Autodesk Inventor part; units mm, degrees
ref_plane "YZ Plane" through (0, 0, 0) normal (1, 0, 0) x (0, 1, 0)
ref_plane "XZ Plane" through (0, 0, 0) normal (0, 1, 0) x (-1, 0, 0)
ref_plane "XY Plane" through (0, 0, 0) normal (0, 0, 1) x (1, 0, 0)
sketch "Sketch1" plane through (0, 0, 0) normal (0, 0, 1) x (1, 0, 0)
  circle A0 centre (0, 0) radius 20
  circle A1 centre (0, 0) radius 23
  dimension "d0" = 40
  dimension "d1" = 46
extrude "Extrusion1" add sketch "Sketch1" along normal mid plane 520
sketch "Sketch2" plane through (0, 0, 0) normal (1, 0, 0) x (0, 1, 0)
  line L0 (0, 280) -> (0, -280)
  line L1 (-280, 0) -> (280, 0)
  point P0 (0, 0)
  point P1 (0, 200)
  point P2 (0, 0)
  point P3 (0, -200)
  dimension "d4" = 200
  dimension "d5" = 200
hole "Hole1" at (0, 0, 200) at (0, 0, 0) at (0, 0, -200) direction (-1, 0, 0) diameter 4.5 end through all
sketch "Sketch3" plane through (0, 0, 0) normal (1, 0, 0) x (0, 1, 0)
  line L0 (23, -240) -> (7, -240)
  line L1 (7, -240) -> (7, 240)
  line L2 (7, 240) -> (23, 240)
  line L3 (23, 240) -> (23, -240)
  line L4 (23, 260) -> (-23, 260)
  line L5 (-23, -260) -> (23, -260)
  line L6 (0, 350) -> (0, -350)
  point P0 (0, 0)
  dimension "d13" = 20
  dimension "d14" = 20
  dimension "d15" = 7
extrude "Extrusion2" cut sketch "Sketch3" along normal through all both and the other way through all
fillet "Fillet1" radius 2 4 edges at (20.3219, 7, -240) (-20.3219, 7, -240) (20.3219, 7, 240) (-20.3219, 7, 240)
properties part number "Pancake_Tilt Pipe" material "PVC-Piping"
For this review, take the finished solid that the model builds, in its own axes (mm). A direction names the side the tool comes from. Give positions to 0.01 mm unless a question says otherwise; leave off trailing zeros. Loops run counter-clockwise (first coordinate to the right, second up) from the corner with the lowest first, then second, coordinate; pieces in that order, holes last. Notation, with made-up numbers: (10.25, -30.5) - (43.25, -30.5) arc R19 cw to (43.25, 4.5) - close; hole circle Ø10 at (65.25, 58). An arc over 180 degrees is marked (long way). Write each question's results on one line, items separated by ' | '.
(1) Take a section at D-D (z = 215.5). Give the boundary of the cut face in (x, y) (3 decimals), then the cut area to 3 significant figures.
Conclusion:
outline: (-21.909, 7) arc R23 ccw (long way) to (21.909, 7) - (18.735, 7) arc R20 cw (long way) to (-18.735, 7) - close | area: 245 mm^2
(2) Draft analysis for pull direction X (two halves, no side actions). For faces 1 (the cylindrical face through (-4.336, -19.524, 3.64)), 2 (the flat face through (-7, 19, -260)), 3 (the cylindrical face through (-2.994, -22.804, -3.64)), state which applies: +X half, -X half, draft (parallel to the pull), parting line (faces both ways), or undercut.
Conclusion:
face 1: undercut | face 2: draft | face 3: parting line
(3) Take a section at C-C (y = -10). Give the boundary of the cut face in (x, z), then the cut area to 3 significant figures.
Conclusion:
outline: (-20.71, -260) - (-17.32, -260) - (-17.32, 260) - (-20.71, 260) - close; (17.32, -260) - (20.71, -260) - (20.71, 260) - (17.32, 260) - close | area: 3,530 mm^2
(4) For pin 1 Ø1 at (x, z) = (-21, 16) entering from +Y; pin 2 Ø7 at (x, y) = (-9.5, 12.5) entering from -Z; pin 3 Ø12 at (x, z) = (2.5, -156.5) entering from +Y; pin 4 Ø3 at (x, z) = (-17, 75.5) entering from +Y, all flat-tipped, find the tip position at first contact; note any pin that passes through.
Conclusion:
pin 1: y = 7 | pin 2: through | pin 3: y = -18.1 | pin 4: y = -7.6
(5) Take a section at B-B (y = 14.5). Give the boundary of the cut face in (x, z), then the cut area to 3 significant figures.
Conclusion:
outline: (-17.85, -260) - (-13.77, -260) - (-13.77, -240) - (-17.85, -240) - close; (-17.85, 240) - (-13.77, 240) - (-13.77, 260) - (-17.85, 260) - close; (13.77, -260) - (17.85, -260) - (17.85, -240) - (13.77, -240) - close; (13.77, 240) - (17.85, 240) - (17.85, 260) - (13.77, 260) - close | area: 326 mm^2
(6) Take a section at A-A (x = 0). Give the boundary of the cut face in (y, z), then the cut area to 3 significant figures.
Conclusion:
outline: (-23, -260) - (-20, -260) - (-20, 260) - (-23, 260) - close; (20, -260) - (23, -260) - (23, -240) - (20, -240) - close; (20, 240) - (23, 240) - (23, 260) - (20, 260) - close | area: 1,680 mm^2
(7) For line 1 along X through (y, z) = (-0.5, 62); line 2 along Z through (x, y) = (6.5, 19); line 3 along X through (y, z) = (-9, -42), list the stretches that pass through material, from the lowest coordinate up.
Conclusion:
line 1: -22.99 to -19.99, 19.99 to 22.99 | line 2: -260 to -240, 240 to 260 | line 3: -21.17 to -17.86, 17.86 to 21.17
(8) For faces 4 (the flat face through (-1.7, 20.1, 240)), 5 (the flat face through (-7, 19, 260)), list the 3-axis set-ups (+Z, -Z, +X, -X, +Y, -Y) from which the entire face can be reached by the end or side of a thin tool; tool diameter is ignored.
Conclusion:
face 4: +X, -X, +Y | face 5: +Z, +X, -X, +Y, -Y
